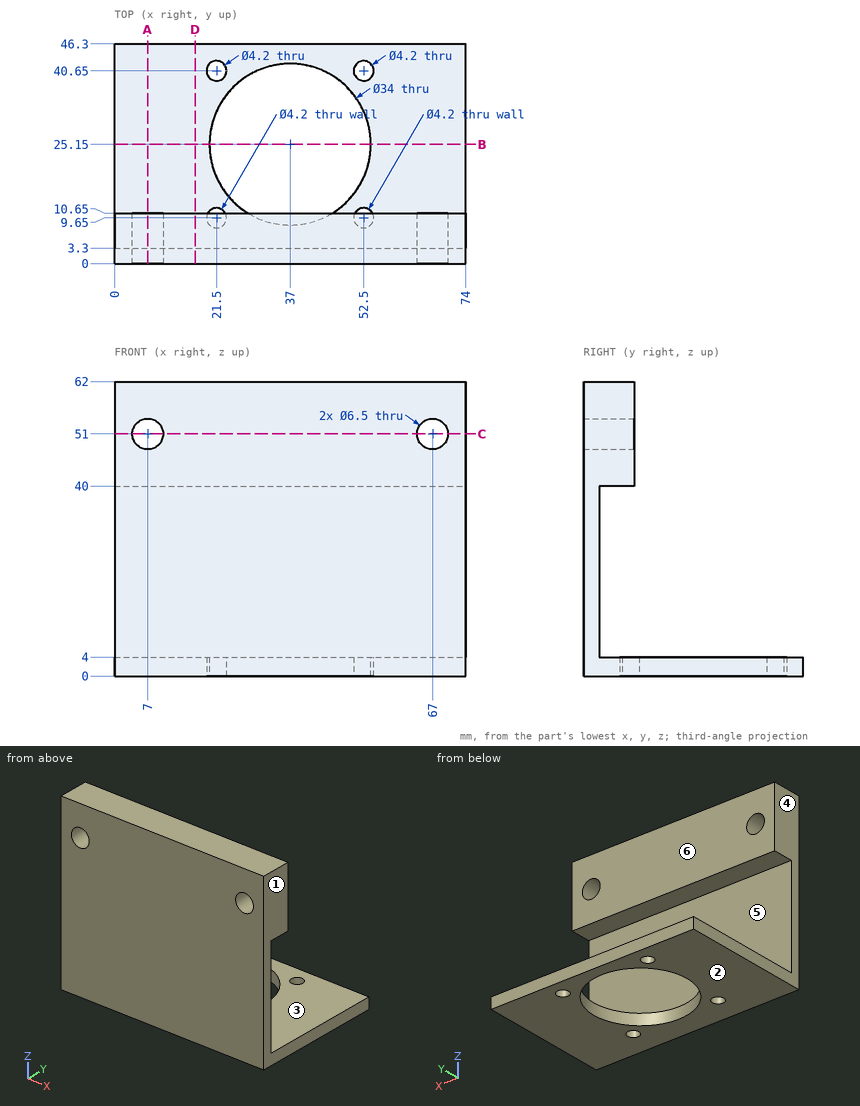
The figure shows three views and two pictorial views of one solid part (mm, origin at its lowest corner). Answer the questions. A direction names the side the tool comes from. Give positions to 0.01 mm unless a question says otherwise; leave off trailing zeros. Write each loop counter-clockwise with the first axis right and the second up, starting at its lowest first coordinate (ties: lowest second). Pieces come first, ordered by that corner, then holes. Notation, with made-up numbers: (61.5, 49) -> (119.5, 49) arc R19 ccw to (119.5, 72) -> close; hole circle Ø10 at (0.25, 71.25). An arc over 180 degrees is marked (long way). Write each question's results on one line, items separated by ' | '.
1. Find section D-D on x = 17. Determine the outline of the cut face in (y, z).
Data:
outline: (0, 0) -> (46.3, 0) -> (46.3, 4) -> (3.3, 4) -> (3.3, 40) -> (10.65, 40) -> (10.65, 62) -> (0, 62) -> close
2. Straight lines are drawn through the part: L1, parallel to Z at x = 7, y = 7.75; L2, parallel to X at y = 5.25, z = 51; L3, parallel to Y at x = 21.5, z = 1.9. For each, find the intervals that lie inside material, in ascending order.
Data:
L1: 0 to 4, 40 to 47.75, 54.25 to 62 | L2: 0 to 3.75, 10.25 to 63.75, 70.25 to 74 | L3: 0 to 7.55, 11.75 to 18.17, 32.13 to 38.55, 42.75 to 46.3
3. Find section C-C on z = 51. Determine the outline of the cut face in (x, y), and give its area (3 significant figures).
Data:
outline: (0, 0) -> (3.75, 0) -> (3.75, 10.65) -> (0, 10.65) -> close; (10.25, 0) -> (63.75, 0) -> (63.75, 10.65) -> (10.25, 10.65) -> close; (70.25, 0) -> (74, 0) -> (74, 10.65) -> (70.25, 10.65) -> close | area: 650 mm^2
4. Find section B-B on y = 25.15. Determine the outline of the cut face in (x, z), and give its area (3 significant figures).
Data:
outline: (0, 0) -> (20, 0) -> (20, 4) -> (0, 4) -> close; (54, 0) -> (74, 0) -> (74, 4) -> (54, 4) -> close | area: 160 mm^2
5. Determine the mould class of the marked faces 1, 2 and 3 for opening direction Z: +Z half, -Z half, draft (parallel to the pull), parting line (faces both ways), or undercut.
Data:
face 1: draft | face 2: -Z half | face 3: undercut
6. Find section A-A on x = 7. Determine the outline of the cut face in (y, z), and give its area (3 significant figures).
Data:
outline: (0, 0) -> (46.3, 0) -> (46.3, 4) -> (3.3, 4) -> (3.3, 40) -> (10.65, 40) -> (10.65, 47.75) -> (0, 47.75) -> close; (0, 54.25) -> (10.65, 54.25) -> (10.65, 62) -> (0, 62) -> close | area: 469 mm^2
7. A tool of negligible diameter and unlimited length cuts with its end or side. For the marked faces 4, 5 and 6, from which of +Z, -Z, +X, -X, +Y, -Y can it reach the whole face along a straight path? Write none if from no direction.
Data:
face 4: +Z, -Z, -X, +Y, -Y | face 5: +X, -X, +Y | face 6: +Z, +X, -X, +Y
8. Each of these flat-tipped pins is pushed along its axis until it touches: pin 1 Ø2.5 at (x, y) = (52.5, 40.65) entering from -Z; pin 2 Ø1.5 at (x, y) = (58, 13) entering from +Z; pin 3 Ø3.5 at (x, y) = (21.5, 9.65) entering from -Z; pin 4 Ø8 at (x, z) = (41.5, 46.5) entering from +Y. Where does it stop, or does it pass through?
Data:
pin 1: through | pin 2: z = 4 | pin 3: z = 40 | pin 4: y = 10.65
